Verification items for the finished model (mm, model axes). Face numbers are marked on the shaded views. A direction names the side the tool comes from. Coordinates: 2 decimals unless noted, no trailing zeros. Order: outer loops, then holes, each group sorted by start corner. A loop starts at its lowest first (then second) coordinate and runs counter-clockwise, first axis right, second up. Notation, with made-up numbers: (38.25, -21.75) -> (48.25, -21.75) arc R27 cw to (48.25, -1.75) -> close; hole circle Ø4 at (73, 64.5). An arc over 180 degrees is marked (long way). Write item = value, one per line. Start each with the question number.
1. Thickness scan on line 1 along X through (y, z) = (61, -1.75); line 2 along Z through (x, y) = (-2.5, 65.5); line 3 along Z through (x, y) = (2.25, 61). Record the ranges inside material, lowest first. Write a range as from..to.
2. Cross-section at A-A on y = 62.5. Record the cut outline in (x, z).
3. Set-up check for the marked faces 1, 2 and 3: record each of +Z, -Z, +X, -X, +Y, -Y from which the full face is reachable in a straight line by a thin tool's end or side.
4. Go/stop test with a flat-tipped pin: P1, Ø1, axis at x = 2.5, y = 56.5, coming from the +Z side. Record where the tip stops, or that it passes through.
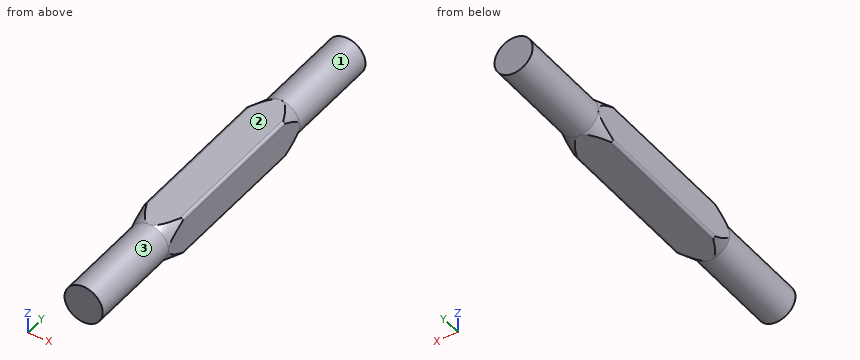
Autodesk Inventor part; units mm, degrees
ref_plane "Plano de trabajo1" through (0, 18, 0) normal (0, 1, 0) x (-1, 0, 0)
ref_plane "YZ Plane" through (0, 0, 0) normal (1, 0, 0) x (0, 1, 0)
ref_plane "XY Plane" through (0, 0, 0) normal (0, 0, 1) x (1, 0, 0)
sketch "Boceto1" plane through (0, 0, 0) normal (0, 1, 0) x (-1, 0, 0)
  circle A0 centre (0, 0) radius 3.5
  dimension "d0" = 7
extrude "Extrusión1" add sketch "Boceto1" along normal blind 72
ref_plane "Plano de trabajo1" through (0, 18, 0) normal (0, 1, 0) x (-1, 0, 0)
sketch "Boceto3" plane through (0, 18, 0) normal (0, 1, 0) x (-1, 0, 0)
  line L0 (-3.5, 0) -> (-3.5, -3.5)
  line L1 (-3.5, -3.5) -> (0, -3.5)
  line L2 (-3.5, -3.5) -> (3.5, -3.5)
  line L3 (3.5, -3.5) -> (3.5, 3.5)
  line L4 (3.5, 3.5) -> (-3.5, 3.5)
  line L5 (-3.5, 3.5) -> (-3.5, -3.5)
  point P0 (0, 0)
  dimension "d26" = 3.5
  dimension "d27" = 3.5
  dimension "d28" = 7
  dimension "d29" = 7
extrude "Extrusión3" add sketch "Boceto3" along normal blind 36
sketch "Boceto4" plane through (0, 0, 0) normal (1, 0, 0) x (0, 1, 0)
  line L0 (0, 0) -> (18, 0)
  line L1 (18, 0) -> (18, 3.5)
  line L2 (23, 5) -> (18, 3.5)
  line L3 (18, 0) -> (54, 0)
  line L4 (54, 0) -> (54, 3.5)
  line L5 (49, 5) -> (54, 3.5)
  line L6 (23, 5) -> (24.5315, 10.105)
  line L7 (24.5315, 10.105) -> (47.4685, 10.105)
  line L8 (18, 3.5) -> (7.2687, 12.5016)
  line L9 (7.2687, 12.5016) -> (61.5507, 12.5016)
  line L10 (61.5507, 12.5016) -> (54, 3.5)
  line L11 (49, 5) -> (47.4685, 10.105)
  dimension "d31" = 18
  dimension "d32" = 3.5
  dimension "d36" = 3.5
revolve "Revolución2" cut sketch "Boceto4" angle 360 about axis through (0, 0, 0) along (0, 1, 0) contours L8 L9 L10 L5 L11 L7 L6 L2
fillet "Empalme1" radius 0.5 4 edges at (3.5, 36, 3.5) (-3.5, 36, 3.5) (3.5, 36, -3.5) (-3.5, 36, -3.5)
thread "Rosca1"
thread "Rosca2"
properties material "Acero"
Worked out:
q1.line_1 = -3.03..3.03
q1.line_2 = -2.45..2.45
q1.line_3 = -2.68..2.68
q2.outline = circle Ø7 at (0, 0)
q3.face_1 = +Y
q3.face_2 = +Z, +X, -X, +Y, -Y
q3.face_3 = -Y
q4.P1 = 2.87
